from build123d import *

# Parameters (mm, degrees)
SKETCH2_W           = 72
SKETCH2_H           = 43
BOSS_EXTRUDE1_DEPTH = 1.5
SKETCH3_R           = 1.4
CUT_EXTRUDE1_DEPTH  = 84.876397157
SKETCH4_W           = 62.5
SKETCH4_H           = 40
BOSS_EXTRUDE2_DEPTH = 3
SKETCH4_2_W         = 62.5
SKETCH4_2_H         = 40
BOSS_EXTRUDE3_DEPTH = 3.5
SKETCH8_W           = 58.989740066
SKETCH8_H           = 32.879527249
CUT_EXTRUDE2_DEPTH  = 0.5


with BuildPart() as part:
    # Sketch2 → Boss-Extrude1 (new body)
    with BuildSketch(Plane(origin=(0, 0, 0), x_dir=(1, 0, 0), z_dir=(0, 1, 0))):
        with Locations((36, 21.5)):
            Rectangle(SKETCH2_W, SKETCH2_H)
    extrude(amount=BOSS_EXTRUDE1_DEPTH)

    # Sketch3 → Cut-Extrude1 (cut, through all)
    with BuildSketch(Plane(origin=(0, 1.5, 0), x_dir=(1, 0, 0), z_dir=(0, 1, 0))):
        with Locations(Location((2, 41, 0), (0, 0, 270))):
            Circle(SKETCH3_R)
        with Locations(Location((70, 41, 0), (0, 0, 270))):
            Circle(SKETCH3_R)
        with Locations(Location((2, 2, 0), (0, 0, 270))):
            Circle(SKETCH3_R)
        with Locations(Location((70, 2, 0), (0, 0, 270))):
            Circle(SKETCH3_R)
    extrude(amount=-CUT_EXTRUDE1_DEPTH, mode=Mode.SUBTRACT)

    # Sketch4 → Boss-Extrude2 (add)
    with BuildSketch(Plane(origin=(0, 1.5, 0), x_dir=(1, 0, 0), z_dir=(0, 1, 0))):
        with Locations((36.25, 20.7)):
            Rectangle(SKETCH4_W, SKETCH4_H)
    extrude(amount=BOSS_EXTRUDE2_DEPTH)

    # Sketch4_2 → Boss-Extrude3 (add)
    with BuildSketch(Plane(origin=(0, 1.5, 0), x_dir=(1, 0, 0), z_dir=(0, 1, 0))):
        with Locations((36.25, 20.7)):
            Rectangle(SKETCH4_2_W, SKETCH4_2_H)
    extrude(amount=-BOSS_EXTRUDE3_DEPTH)

    # Sketch8 → Cut-Extrude2 (cut)
    with BuildSketch(Plane(origin=(0, 4.5, 0), x_dir=(1, 0, 0), z_dir=(0, 1, 0))):
        with Locations((36.379910504, 22.622462852)):
            Rectangle(SKETCH8_W, SKETCH8_H)
    extrude(amount=-CUT_EXTRUDE2_DEPTH, mode=Mode.SUBTRACT)


solid = part.part
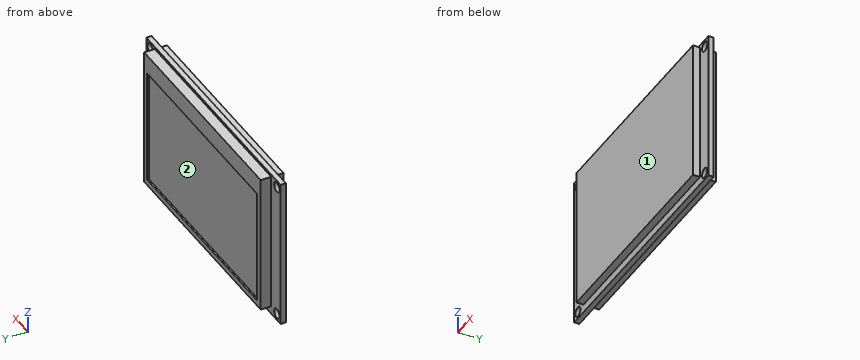
CAD build for the part. Positions are in the model's coordinates, mm. Face numbers are marked on the shaded views. Coordinates: 2 decimals unless noted, no trailing zeros. Write each loop counter-clockwise with the first axis right and the second up, starting at its lowest first coordinate (ties: lowest second). Pieces come first, ordered by that corner, then holes. Notation, with made-up numbers: M -23.75,34.5 L 0.25,34.5 A21 ccw 0.25,39.5 Z; hole C -12,33.5 d11. An arc over 180 degrees is marked long. Return JSON: item names as keys, results as strings.
Item 1: Slice it at B-B, the plane z = -2. Write the cut outline in (x, y), and give its area (3 significant figures).
Findings below:
{"outline": "M 0,0 L 0.6,0 L 0.6,1.5 L 0,1.5 Z; M 3.4,0 L 5,0 L 5,-2 L 67.5,-2 L 67.5,0 L 68.6,0 L 68.6,1.5 L 67.5,1.5 L 67.5,4.5 L 5,4.5 L 5,1.5 L 3.4,1.5 Z; M 71.4,0 L 72,0 L 72,1.5 L 71.4,1.5 Z", "area": "412 mm2"}
Item 2: Slice it at C-C, the plane z = -21. Write the cut outline in (x, y), and give its area (3 significant figures).
Findings below:
{"outline": "M 0,0 L 5,0 L 5,-2 L 67.5,-2 L 67.5,0 L 72,0 L 72,1.5 L 67.5,1.5 L 67.5,4.5 L 65.87,4.5 L 65.87,4 L 6.89,4 L 6.89,4.5 L 5,4.5 L 5,1.5 L 0,1.5 Z", "area": "391 mm2"}
Item 3: Drop flat-ended pins along their axis: pin 1 Ø3 at (x, z) = (70, -41) entering from +Y; pin 2 Ø16.5 at (x, z) = (34.5, -28) entering from +Y; pin 3 Ø1.5 at (x, y) = (29.5, 2.5) entering from +Z. Give the stop position or say it passes through.
Findings below:
{"pin 1": "stops at y = 1.5", "pin 2": "stops at y = 4", "pin 3": "stops at z = -0.7"}
Item 4: Probe line 1 (X direction, y = 0.85, z = -41); line 2 (Z direction, x = 70, y = 1.15); line 3 (Z direction, x = 16.5, y = 3.25). List the from-to ranges inside material, lowest first. Write a range as from..to.
Findings below:
{"line 1": "x = 0..0.6, 3.4..68.6, 71.4..72", "line 2": "z = -43..-42.4, -39.6..-3.4, -0.6..0", "line 3": "z = -40.7..-0.7"}
Item 5: Slice it at A-A, the plane x = 70. Write the cut outline in (y, z).
Findings below:
{"outline": "M 0,-43 L 1.5,-43 L 1.5,-42.4 L 0,-42.4 Z; M 0,-39.6 L 1.5,-39.6 L 1.5,-3.4 L 0,-3.4 Z; M 0,-0.6 L 1.5,-0.6 L 1.5,0 L 0,0 Z"}
Item 6: Two-plate mould, pull along X, no slides. Class the marked faces 1 and 2: +X half, -X half, draft (parallel to the pull), parting line (faces both ways), or undercut.
Findings below:
{"face 1": "draft", "face 2": "undercut"}
